from build123d import *

# Parameters (mm, degrees)
BASE_FLANGE1_DEPTH            = 2
EDGE_FLANGE1_STRIP_W          = 16
EDGE_FLANGE1_STRIP_H          = 2
EDGE_FLANGE1_STRIP_CUT_DEPTH  = 363.829009869
EDGE_FLANGE1_RELIEF_W         = 17
EDGE_FLANGE1_RELIEF_H         = 1
EDGE_FLANGE1_RELIEF_CUT_DEPTH = 2
EDGE_FLANGE1_DEPTH            = 363.829009869
EDGE_FLANGE2_STRIP_W          = 16
EDGE_FLANGE2_STRIP_H          = 2
EDGE_FLANGE2_STRIP_CUT_DEPTH  = 894
EDGE_FLANGE2_DEPTH            = 894
EDGE_FLANGE3_STRIP_W          = 16
EDGE_FLANGE3_STRIP_H          = 2
EDGE_FLANGE3_STRIP_CUT_DEPTH  = 894
EDGE_FLANGE3_DEPTH            = 894
EDGE_FLANGE4_START            = 1915.177869048
EDGE_FLANGE4_DEPTH            = 394.75629901
EDGE_FLANGE4_2_DEPTH          = 1
EDGE_FLANGE4_START_2          = 1916.177869048
EDGE_FLANGE4_3_DEPTH          = 393.75629901
SKETCH20_W                    = 43
SKETCH20_H                    = 34
CUT_EXTRUDE1_DEPTH            = 10
SKETCH21_W                    = 43
SKETCH21_H                    = 34
CUT_EXTRUDE2_DEPTH            = 10
SKETCH22_R                    = 4.25
CUT_EXTRUDE3_DEPTH            = 10
SKETCH23_R                    = 4.25
CUT_EXTRUDE4_DEPTH            = 10


# Read off the part's stored shape, not the designer's step: Edge-Flange4
# Sheet-metal steps are written as plain solids
with BuildPart() as part:
    # Sketch1 → Base-Flange1 (new body)
    with BuildSketch(Plane(origin=(0, 0, 0), x_dir=(1, 0, 0), z_dir=(0, 1, 0))):
        with BuildLine():
            Line((-2530.611542613, -1415.934168058), (-2166.782532744, -1415.934168058))
            Line((-2166.782532744, -1415.934168058), (-2166.782532744, -2315.934168058))
            Line((-2166.782532744, -2315.934168058), (-3066.782532744, -2315.934168058))
            Line((-3066.782532744, -2315.934168058), (-3066.782532744, -1916.177869048))
            ThreePointArc((-3066.782532744, -1916.177869048), (-2760.872899609, -1706.596670078), (-2530.611542613, -1415.934168058))
        make_face()
    extrude(amount=-BASE_FLANGE1_DEPTH)

    # Edge-Flange1 strip (across the edge) → Edge-Flange1 strip cut (cut)
    with BuildSketch(Plane(origin=(-2166.782532744, 0, 1415.934168058), x_dir=(0, 0, 1), z_dir=(-1, 0, 0))):
        with Locations((-2, -1)):
            Rectangle(EDGE_FLANGE1_STRIP_W, EDGE_FLANGE1_STRIP_H)
    extrude(amount=EDGE_FLANGE1_STRIP_CUT_DEPTH, mode=Mode.SUBTRACT)

    # Edge-Flange1 relief (on the sheet) → Edge-Flange1 relief cut (cut)
    with BuildSketch(Plane(origin=(-2166.782532744, 0, 1421.934168058), x_dir=(0, 0, 1), z_dir=(0, 1, 0))):
        with Locations((-7.5, -364.329009869)):
            Rectangle(EDGE_FLANGE1_RELIEF_W, EDGE_FLANGE1_RELIEF_H)
    extrude(amount=-EDGE_FLANGE1_RELIEF_CUT_DEPTH, mode=Mode.SUBTRACT)

    # Edge-Flange1 section (across the edge) → Edge-Flange1 (add)
    with BuildSketch(Plane(origin=(-2166.782532744, 0, 1415.934168058), x_dir=(0, 0, 1), z_dir=(-1, 0, 0))):
        with BuildLine():
            Line((0, 4), (0, 38))
            Line((0, 38), (2, 38))
            Line((2, 38), (2, 4))
            ThreePointArc((2, 4), (3.171572875, 1.171572875), (6, 0))
            Line((6, 0), (6, -2))
            ThreePointArc((6, -2), (1.757359313, -0.242640687), (0, 4))
        make_face()
    extrude(amount=EDGE_FLANGE1_DEPTH)

    # Edge-Flange2 strip (across the edge) → Edge-Flange2 strip cut (cut)
    with BuildSketch(Plane(origin=(-2166.782532744, 0, 2315.934168058), x_dir=(-1, 0, 0), z_dir=(0, 0, -1))):
        with Locations((-2, -1)):
            Rectangle(EDGE_FLANGE2_STRIP_W, EDGE_FLANGE2_STRIP_H)
    extrude(amount=EDGE_FLANGE2_STRIP_CUT_DEPTH, mode=Mode.SUBTRACT)

    # Edge-Flange2 section (across the edge) → Edge-Flange2 (add)
    with BuildSketch(Plane(origin=(-2166.782532744, 0, 2315.934168058), x_dir=(-1, 0, 0), z_dir=(0, 0, -1))):
        with BuildLine():
            Line((0, 4), (0, 38))
            Line((0, 38), (2, 38))
            Line((2, 38), (2, 4))
            ThreePointArc((2, 4), (3.171572875, 1.171572875), (6, 0))
            Line((6, 0), (6, -2))
            ThreePointArc((6, -2), (1.757359313, -0.242640687), (0, 4))
        make_face()
    extrude(amount=EDGE_FLANGE2_DEPTH)

    # Edge-Flange3 strip (across the edge) → Edge-Flange3 strip cut (cut)
    with BuildSketch(Plane(origin=(-3066.782532744, 0, 2315.934168058), x_dir=(0, 0, -1), z_dir=(1, 0, 0))):
        with Locations((-2, -1)):
            Rectangle(EDGE_FLANGE3_STRIP_W, EDGE_FLANGE3_STRIP_H)
    extrude(amount=EDGE_FLANGE3_STRIP_CUT_DEPTH, mode=Mode.SUBTRACT)

    # Edge-Flange3 section (across the edge) → Edge-Flange3 (add)
    with BuildSketch(Plane(origin=(-3066.782532744, 0, 2315.934168058), x_dir=(0, 0, -1), z_dir=(1, 0, 0))):
        with BuildLine():
            Line((0, 4), (0, 38))
            Line((0, 38), (2, 38))
            Line((2, 38), (2, 4))
            ThreePointArc((2, 4), (3.171572875, 1.171572875), (6, 0))
            Line((6, 0), (6, -2))
            ThreePointArc((6, -2), (1.757359313, -0.242640687), (0, 4))
        make_face()
    extrude(amount=EDGE_FLANGE3_DEPTH)

    # Edge-Flange4 outline → Edge-Flange4 (cut)
    with BuildSketch(Plane.XY.offset(EDGE_FLANGE4_START)):
        with BuildLine():
            ThreePointArc((-3060.782532744, -2), (-3063.232022487, -1.477225575), (-3065.254668699, 0))
            Line((-3065.254668699, 0), (-3066.782532744, 0))
            Line((-3066.782532744, 0), (-3066.782532744, -2))
            Line((-3066.782532744, -2), (-3060.782532744, -2))
        make_face()
    extrude(amount=EDGE_FLANGE4_DEPTH, mode=Mode.SUBTRACT)

    # Edge-Flange4 2 outline → Edge-Flange4 2 (cut)
    with BuildSketch(Plane.XY.offset(EDGE_FLANGE4_START)):
        with BuildLine():
            Line((-3059.782532744, 0), (-3065.254668699, 0))
            ThreePointArc((-3065.254668699, 0), (-3063.232022487, -1.477225575), (-3060.782532744, -2))
            Line((-3060.782532744, -2), (-3059.782532744, -2))
            Line((-3059.782532744, -2), (-3059.782532744, 0))
        make_face()
    extrude(amount=EDGE_FLANGE4_2_DEPTH, mode=Mode.SUBTRACT)

    # Edge-Flange4 3 outline → Edge-Flange4 3 (add)
    with BuildSketch(Plane.XY.offset(EDGE_FLANGE4_START_2)):
        with BuildLine():
            Line((-3064.782532744, 38), (-3066.782532744, 38))
            Line((-3066.782532744, 38), (-3066.782532744, 4))
            ThreePointArc((-3066.782532744, 4), (-3066.387566898, 1.859067461), (-3065.254668699, 0))
            Line((-3065.254668699, 0), (-3060.782532744, 0))
            ThreePointArc((-3060.782532744, 0), (-3063.610959869, 1.171572875), (-3064.782532744, 4))
            Line((-3064.782532744, 4), (-3064.782532744, 38))
        make_face()
    extrude(amount=EDGE_FLANGE4_3_DEPTH)

    # Sketch20 → Cut-Extrude1 (cut)
    with BuildSketch(Plane.ZY.offset(3066.782532744)):
        with Locations((1937.677869048, 21)):
            Rectangle(SKETCH20_W, SKETCH20_H)
    extrude(amount=-CUT_EXTRUDE1_DEPTH, mode=Mode.SUBTRACT)

    # Sketch21 → Cut-Extrude2 (cut)
    with BuildSketch(Plane(origin=(0, 0, 1415.934168058), x_dir=(-1, 0, 0), z_dir=(0, 0, -1))):
        with Locations((2509.111542613, 21)):
            Rectangle(SKETCH21_W, SKETCH21_H)
    extrude(amount=-CUT_EXTRUDE2_DEPTH, mode=Mode.SUBTRACT)

    # Sketch22 → Cut-Extrude3 (cut)
    with BuildSketch(Plane(origin=(0, 0, 1415.934168058), x_dir=(-1, 0, 0), z_dir=(0, 0, -1))):
        with Locations(Location((2200.932532744, 21, 0), (0, 0, 90))):
            Circle(SKETCH22_R)
        with Locations(Location((2325.932532744, 21, 0), (0, 0, 90))):
            Circle(SKETCH22_R)
        with Locations(Location((2450.932532744, 21, 0), (0, 0, 90))):
            Circle(SKETCH22_R)
    extrude(amount=-CUT_EXTRUDE3_DEPTH, mode=Mode.SUBTRACT)

    # Sketch23 → Cut-Extrude4 (cut)
    with BuildSketch(Plane.ZY.offset(3066.782532744)):
        with Locations((2281.784168058, 21)):
            Circle(SKETCH23_R)
        with Locations((2156.784168058, 21)):
            Circle(SKETCH23_R)
        with Locations((2031.784168058, 21)):
            Circle(SKETCH23_R)
    extrude(amount=-CUT_EXTRUDE4_DEPTH, mode=Mode.SUBTRACT)


solid = part.part
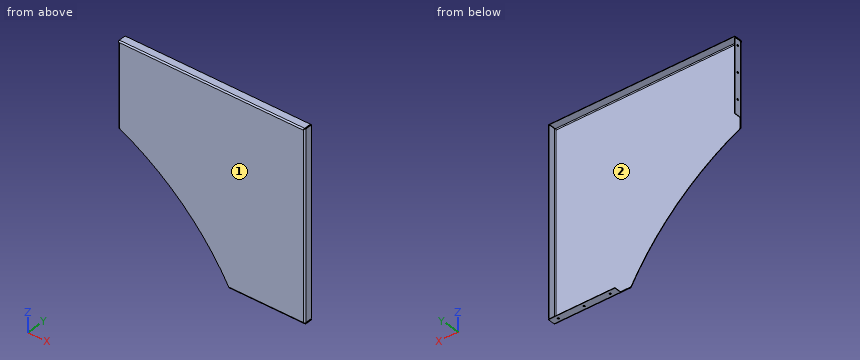
Model file for the job. Use its own axes, mm. Face numbers are marked on the shaded views. Give positions to 0.01 mm unless a question says otherwise; leave off trailing zeros. Order: outer loops, then holes, each group sorted by start corner. A loop starts at its lowest first (then second) coordinate and runs counter-clockwise, first axis right, second up. Notation, with made-up numbers: (29, 62.25) - (42, 62.25) arc R5 cw to (42, 69.25) - close; hole circle Ø4 at (38.25, 61.5). An arc over 180 degrees is marked (long way). One line per item, written item: value.
Item 1: Wall check: line 1 (X direction, y = 21, z = 1416); line 2 (X direction, y = 6, z = 2011); line 3 (Z direction, x = -2277, y = 32). Give the ranges that are in metal, low to high.
Response values:
line 1: -2487.61 to -2455.18, -2446.68 to -2330.18, -2321.68 to -2205.18, -2196.68 to -2166.78
line 2: -3066.78 to -3064.78, -2168.78 to -2166.78
line 3: 1415.93 to 1417.93, 2313.93 to 2315.93
Item 2: Slice it at D-D (x = -2918.5). List the corners of the cut face in (y, z), then the cut area to 3 significant figures.
Response values:
outline: (-2, 1831.37) - (0, 1831.37) - (0, 2309.93) arc R4 cw to (4, 2313.93) - (38, 2313.93) - (38, 2315.93) - (4, 2315.93) arc R6 ccw to (-2, 2309.93) - close
area: 1,040 mm2
Item 3: Slice it at C-C (z = 2130). List the corners of the cut face in (x, y).
Response values:
outline: (-3066.78, 4) arc R6 ccw to (-3060.78, -2) - (-2172.78, -2) arc R6 ccw to (-2166.78, 4) - (-2166.78, 38) - (-2168.78, 38) - (-2168.78, 4) arc R4 cw to (-2172.78, 0) - (-3060.78, 0) arc R4 cw to (-3064.78, 4) - (-3064.78, 38) - (-3066.78, 38) - close
Item 4: Pin check, flat tips, straight feed: pin 1 Ø0.6 at (x, y) = (-3066, 27.5) entering from -Z; pin 2 Ø1.8 at (y, z) = (0.5, 1420) entering from -X; pin 3 Ø1 at (x, z) = (-2514, 1417.5) entering from +Y; pin 4 Ø10 at (y, z) = (2.5, 1862) entering from +X. Stop position of each tip, or through.
Response values:
pin 1: z = 1959.18
pin 2: x = -2533.38
pin 3: y = 4
pin 4: x = -2166.78
Item 5: Slice it at A-A (y = 32). List the corners of the cut face in (x, z).
Response values:
outline: (-3066.78, 1959.18) - (-3064.78, 1959.18) - (-3064.78, 2309.93) - (-3066.78, 2309.93) - close; (-3066.78, 2313.93) - (-2172.78, 2313.93) - (-2172.78, 2315.93) - (-3066.78, 2315.93) - close; (-2487.61, 1415.93) - (-2166.78, 1415.93) - (-2166.78, 1417.93) - (-2487.61, 1417.93) - close; (-2168.78, 1421.93) - (-2166.78, 1421.93) - (-2166.78, 2315.93) - (-2168.78, 2315.93) - close
Item 6: Two-plate mould, pull along X, no slides. Class the marked faces 1 and 2: released by +X, released by -X, zero draft, split by the parting line, or undercut.
Response values:
face 1: zero draft
face 2: undercut
Item 7: Slice it at B-B (x = -2225.5). List the corners of the cut face in (y, z).
Response values:
outline: (-2, 1421.93) arc R6 ccw to (4, 1415.93) - (38, 1415.93) - (38, 1417.93) - (4, 1417.93) arc R4 cw to (0, 1421.93) - (0, 2309.93) arc R4 cw to (4, 2313.93) - (38, 2313.93) - (38, 2315.93) - (4, 2315.93) arc R6 ccw to (-2, 2309.93) - close
